Source: CAD feature listing. Evaluate the final solid. Frame: model axes, mm. A direction names the side the tool comes from. Round coordinates to 2 decimals unless told otherwise and drop trailing zeros. Loops run counter-clockwise (first coordinate to the right, second up) from the corner with the lowest first, then second, coordinate; pieces in that order, holes last. Notation, with made-up numbers: (26.5, 35) -> (39.5, 35) arc R26 cw to (39.5, 55) -> close; hole circle Ø1 at (-30.5, -28.5). An arc over 180 degrees is marked (long way). Return JSON: item names as keys, results as strings. Group by question number.
```python
from build123d import *

# Parameters (mm, degrees)
EXTRUDE_1_DEPTH = 10
SKETCH_2_R      = 15
EXTRUDE_2_DEPTH = 15
SKETCH_3_W      = 5
SKETCH_3_H      = 10
EXTRUDE_3_DEPTH = 30


with BuildPart() as part:
    # ｽｹｯﾁ1 → ﾎﾞｽ - 押し出し1 (new body)
    with BuildSketch(Plane.XY):
        with BuildLine():
            Line((0, 0), (30, 0))
            Line((30, 0), (30, 20))
            ThreePointArc((30, 20), (15, 35), (0, 20))
            Line((0, 20), (0, 0))
        make_face()
    extrude(amount=EXTRUDE_1_DEPTH)

    # ｽｹｯﾁ2 → ﾎﾞｽ - 押し出し2 (add)
    with BuildSketch(Plane.XY.offset(10)):
        with Locations((15, 15)):
            Circle(SKETCH_2_R)
    extrude(amount=EXTRUDE_2_DEPTH)

    # ｽｹｯﾁ3 → ﾎﾞｽ - 押し出し3 (add)
    with BuildSketch(Plane.XY.offset(25)):
        with Locations((15, 15)):
            Rectangle(SKETCH_3_W, SKETCH_3_H)
    extrude(amount=EXTRUDE_3_DEPTH)


solid = part.part
```
(1) Set-up query: faces 1 (the face through (3, 6, 17)), 2 (the face through (17.5, 15, 40)), 3 (the face through (15, 20, 40)), 4 (the face through (12.5, 15, 40)), 5 (the face through (27, 3, 10)). Return all of +Z, -Z, +X, -X, +Y, -Y with unobstructed straight access to the full face (end or side cutting, diameter ignored); none if empty.
(2) Cut plane B-B (y = 25.5). Return loops of the section in (x, z).
(3) Cut plane C-C (z = 45.5). Return loops of the section in (x, y).
(4) Pin query (flat end, axial travel): pin 1 (12 mm diameter, centred on y = 7.5, z = 25.5, fed in from -X); pin 2 (7.5 mm diameter, centred on x = 25.5, y = 8, fed in from +Z); pin 3 (1 mm diameter, centred on x = 4.5, z = 25, fed in from +Y); pin 4 (10 mm diameter, centred on x = 23, z = 34, fed in from -Y). Return the tip coordinate at first contact, or that it passes through.
(5) Cut plane D-D (z = 3.5). Return loops of the section in (x, y).
(6) Cut plane A-A (x = 24). Return loops of the section in (y, z), and give its area (3 significant figures).
(7) Ray query, line 1 (Z direction, x = 25, y = 16); line 2 (Z direction, x = 28, y = 23.5); line 3 (X direction, y = 17, z = 28). Return the intervals inside material, ascending.
Answers follow:
{
 "1": {"face 1": "+Z", "face 2": "+Z, +X, +Y, -Y", "face 3": "+Z, +X, -X, +Y", "face 4": "+Z, -X, +Y, -Y", "face 5": "+Z, +X, -Y"},
 "2": {"outline": "(1.04, 0) -> (28.96, 0) -> (28.96, 10) -> (25.71, 10) -> (25.71, 25) -> (4.29, 25) -> (4.29, 10) -> (1.04, 10) -> close"},
 "3": {"outline": "(12.5, 10) -> (17.5, 10) -> (17.5, 20) -> (12.5, 20) -> close"},
 "4": {"pin 1": "x = 0.08", "pin 2": "z = 25", "pin 3": "y = 26.18", "pin 4": "through"},
 "5": {"outline": "(0, 0) -> (30, 0) -> (30, 20) arc R15 ccw to (0, 20) -> close"},
 "6": {"outline": "(0, 0) -> (32, 0) -> (32, 10) -> (27, 10) -> (27, 25) -> (3, 25) -> (3, 10) -> (0, 10) -> close", "area": "680 mm^2"},
 "7": {"line 1": "0 to 25", "line 2": "0 to 10", "line 3": "12.5 to 17.5"}
}
